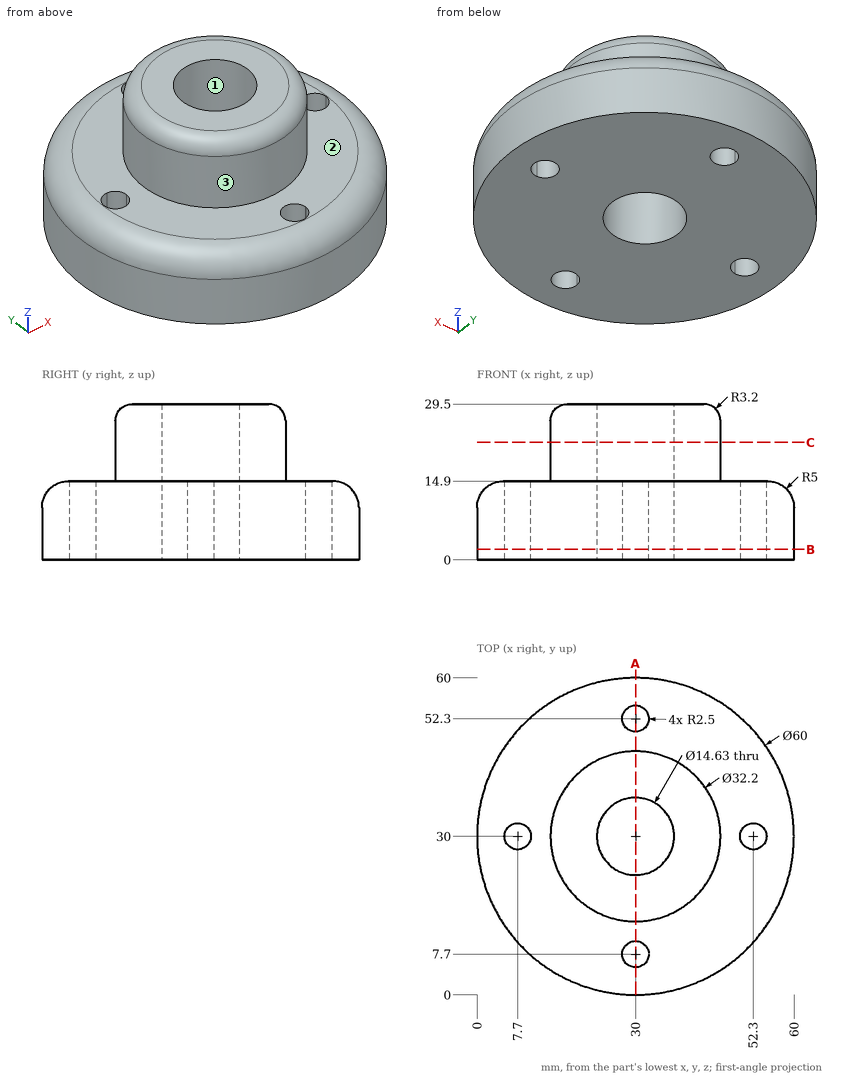
Drawing for the job (mm, zero at the part's lowest x, y, z). Round coordinates to 2 decimals unless told otherwise and drop trailing zeros. Order: outer loops, then holes, each group sorted by start corner. A loop starts at its lowest first (then second) coordinate and runs counter-clockwise, first axis right, second up. Notation, with made-up numbers: (-2.5, 9.25) -> (13.5, 9.25) arc R18 ccw to (13.5, 44.25) -> close; hole circle Ø2 at (-18.75, 27). An arc over 180 degrees is marked (long way). Write item = value, one per line. Start each with the question number.
(1) Cut at B-B, the plane z = 2. List the corners of the cut face in (x, y) (3 decimals).
(2) Probe line 1 (Y direction, x = 30, z = 10.25) (3 decimals); line 2 (Y direction, x = 30, z = 15) (3 decimals); line 3 (Z direction, x = 12, y = 31.5). List the from-to ranges inside material, lowest first. Write a range as [from, to].
(3) Pin check, flat tips, straight feed: P1, Ø8, axis at x = 30.5, z = 11.5, coming from the -Y side; P2, Ø5, axis at x = 40.5, z = 13, coming from the +Y side; P3, Ø8, axis at x = 42.5, z = 21.5, coming from the -Y side. Stop position of each tip, or through.
(4) Cut at C-C, the plane z = 22.25. List the corners of the cut face in (x, y) (3 decimals), then the cut area to 3 significant figures.
(5) Pull direction Y, two halves, no side cores. Call the marked faces 1, 2 and 3: released by +Y, released by -Y, zero draft, split by the parting line, or undercut.
(6) Cut at A-A, the plane x = 30. List the corners of the cut face in (y, z) (3 decimals), then the cut area to 3 significant figures.
Model answer:
q1.outline = circle Ø60 at (30, 30); hole (7.84, 27.504) arc R2.5 ccw to (10.2, 30) arc R2.5 ccw to (7.84, 32.496) arc R2.5 ccw (long way) to start; hole circle Ø14.63 at (30, 30); hole (32.496, 7.84) arc R2.5 ccw (long way) to (32.5, 7.7) arc R2.5 ccw to start; hole (32.496, 52.16) arc R2.5 ccw to (32.5, 52.3) arc R2.5 ccw (long way) to start; hole (52.16, 27.504) arc R2.5 ccw to (54.8, 30) arc R2.5 ccw to (52.16, 32.496) arc R2.5 ccw to start
q2.line_1 = [0.012, 5.2], [10.2, 22.685], [37.315, 49.8], [54.8, 59.988]
q2.line_2 = [13.9, 22.685], [37.315, 46.1]
q2.line_3 = [0, 14.9]
q3.P1 = 0
q3.P2 = 58.51
q3.P3 = 16.33
q4.outline = circle Ø32.2 at (30, 30); hole circle Ø14.63 at (30, 30)
q4.area = 646 mm2
q5.face_1 = undercut
q5.face_2 = zero draft
q5.face_3 = split by the parting line
q6.outline = (0, 0) -> (5.2, 0) -> (5.2, 14.9) -> (5, 14.9) arc R5 ccw to (0, 9.9) -> close; (10.2, 0) -> (22.685, 0) -> (22.685, 29.5) -> (17.1, 29.5) arc R3.2 ccw to (13.9, 26.3) -> (13.9, 14.9) -> (10.2, 14.9) -> close; (37.315, 0) -> (49.8, 0) -> (49.8, 14.9) -> (46.1, 14.9) -> (46.1, 26.3) arc R3.2 ccw to (42.9, 29.5) -> (37.315, 29.5) -> close; (54.8, 0) -> (60, 0) -> (60, 9.9) arc R5 ccw to (55, 14.9) -> (54.8, 14.9) -> close
q6.area = 768 mm2
